```python
from build123d import *

# Parameters (mm, degrees)
BOSS_EXTRUDE1_DEPTH     = 2
BOSS_EXTRUDE2_START     = 2
BOSS_EXTRUDE2_DEPTH     = 2.5
BOSS_EXTRUDE3_START     = 4.5
SKETCH1_6_R             = 3.25
BOSS_EXTRUDE3_DEPTH     = 2
BOSS_EXTRUDE6_DEPTH     = 33.8
BOSS_EXTRUDE7_DEPTH     = 3.8
FILLET1_R               = 2
FILLET2_R               = 2
FILLET3_R               = 0.5
CUT_EXTRUDE1_REACH      = 54.552
CUT_EXTRUDE1_END_RADIUS = 27.541666667
SKETCH6_R               = 3.25


with BuildPart() as part:
    # Sketch1 → Boss-Extrude1 (new body)
    with BuildSketch(Plane(origin=(0, 0, 0), x_dir=(1, 0, 0), z_dir=(0, 1, 0))):
        with BuildLine():
            ThreePointArc((0, 8.25), (-8.25, 0), (0, -8.25))
            Line((0, -8.25), (0, -3.25))
            ThreePointArc((0, -3.25), (-3.25, 0), (0, 3.25))
            Line((0, 3.25), (0, 8.25))
        make_face()
        with BuildLine():
            Line((0, -3.25), (0, -8.25))
            ThreePointArc((0, -8.25), (5.833630945, -5.833630945), (8.25, 0))
            ThreePointArc((8.25, 0), (5.833630945, 5.833630945), (0, 8.25))
            Line((0, 8.25), (0, 3.25))
            ThreePointArc((0, 3.25), (2.298097039, 2.298097039), (3.25, 0))
            ThreePointArc((3.25, 0), (2.298097039, -2.298097039), (0, -3.25))
        make_face()
        with BuildLine():
            Line((0, -8.25), (0, -9.25))
            ThreePointArc((0, -9.25), (9.25, 0), (0, 9.25))
            Line((0, 9.25), (0, 8.25))
            ThreePointArc((0, 8.25), (5.833630945, 5.833630945), (8.25, 0))
            ThreePointArc((8.25, 0), (5.833630945, -5.833630945), (0, -8.25))
        make_face()
        with BuildLine():
            Line((0, -12.5), (22, -12.5))
            ThreePointArc((22, -12.5), (19, 0), (22, 12.5))
            Line((22, 12.5), (0, 12.5))
            Line((0, 12.5), (0, 9.25))
            ThreePointArc((0, 9.25), (9.25, 0), (0, -9.25))
            Line((0, -9.25), (0, -12.5))
        make_face()
        with BuildLine():
            Line((22, -12.5), (30, -12.5))
            Line((30, -12.5), (30, 12.5))
            Line((30, 12.5), (22, 12.5))
            ThreePointArc((22, 12.5), (19, 0), (22, -12.5))
        make_face()
    extrude(amount=BOSS_EXTRUDE1_DEPTH)

    # Sketch1<4> → Boss-Extrude2 (add)
    with BuildSketch(Plane(origin=(0, 0, 0), x_dir=(1, 0, 0), z_dir=(0, 1, 0)).offset(BOSS_EXTRUDE2_START)):
        with BuildLine():
            Line((30, -12.5), (30, 12.5))
            Line((30, 12.5), (0, 12.5))
            Line((0, 12.5), (0, 9.25))
            ThreePointArc((0, 9.25), (9.25, 0), (0, -9.25))
            Line((0, -9.25), (0, -12.5))
            Line((0, -12.5), (30, -12.5))
        make_face()
    extrude(amount=BOSS_EXTRUDE2_DEPTH)

    # Sketch1<6> → Boss-Extrude3 (add)
    with BuildSketch(Plane(origin=(0, 0, 0), x_dir=(1, 0, 0), z_dir=(0, 1, 0)).offset(BOSS_EXTRUDE3_START)):
        with BuildLine():
            Line((30, -12.5), (30, 12.5))
            Line((30, 12.5), (0, 12.5))
            Line((0, 12.5), (0, 8.25))
            ThreePointArc((0, 8.25), (-8.25, 0), (0, -8.25))
            Line((0, -8.25), (0, -12.5))
            Line((0, -12.5), (30, -12.5))
        make_face()
        with Locations(Location((0, 0, 0), (0, 0, 270))):
            Circle(SKETCH1_6_R, mode=Mode.SUBTRACT)
    extrude(amount=BOSS_EXTRUDE3_DEPTH)

    # Sketch1<8> → Boss-Extrude6 (add)
    with BuildSketch(Plane(origin=(0, 0, 0), x_dir=(1, 0, 0), z_dir=(0, 1, 0))):
        with BuildLine():
            Line((22, -12.5), (30, -12.5))
            Line((30, -12.5), (30, 12.5))
            Line((30, 12.5), (22, 12.5))
            ThreePointArc((22, 12.5), (19, 0), (22, -12.5))
        make_face()
    extrude(amount=BOSS_EXTRUDE6_DEPTH)

    # Sketch3 → Boss-Extrude7 (add)
    with BuildSketch(Plane(origin=(0, 33.8, 0), x_dir=(1, 0, 0), z_dir=(0, 1, 0))):
        with BuildLine():
            Line((11, 0), (19, 0))
            ThreePointArc((19, 0), (19.473969858, 5.087552676), (20.879566153, 10))
            Line((20.879566153, 10), (11, 0))
        make_face()
        with BuildLine():
            ThreePointArc((20.879566153, -10), (19.473969858, -5.087552676), (19, 0))
            Line((19, 0), (11, 0))
            Line((11, 0), (20.879566153, -10))
        make_face()
        with BuildLine():
            ThreePointArc((20.879566153, 10), (19.473969858, 5.087552676), (19, 0))
            ThreePointArc((19, 0), (19.473969858, -5.087552676), (20.879566153, -10))
            ThreePointArc((20.879566153, -10), (21.408679185, -11.263939941), (22, -12.5))
            Line((22, -12.5), (30, -12.5))
            Line((30, -12.5), (30, 12.5))
            Line((30, 12.5), (22, 12.5))
            ThreePointArc((22, 12.5), (21.408679185, 11.263939941), (20.879566153, 10))
        make_face()
    extrude(amount=-BOSS_EXTRUDE7_DEPTH)

    # Fillet1
    fillet1_edges = [part.edges().sort_by_distance(p)[0] for p in [
        (11, 31.9, 0),
    ]]
    fillet(fillet1_edges, radius=FILLET1_R)

    # Fillet2
    fillet2_edges = [part.edges().sort_by_distance(p)[0] for p in [
        (30, 16.9, -12.5),
        (30, 16.9, 12.5),
        (22, 20.15, -12.5),
        (22, 20.15, 12.5),
    ]]
    fillet(fillet2_edges, radius=FILLET2_R)

    # Fillet3
    fillet3_edges = [part.edges().sort_by_distance(p)[0] for p in [
        (0, 2, 8.75),
        (0, 3.25, -9.25),
        (0, 3.25, 9.25),
        (0, 2, -8.75),
        (0, 4.5, -8.75),
        (-8.25, 4.5, 0),
        (0, 4.5, 8.75),
        (-8.25, 2, 0),
    ]]
    fillet(fillet3_edges, radius=FILLET3_R)

    # Cut-Extrude1: up to this cylinder (the profile starts inside it)
    cut_extrude1_end = Plane(origin=(46.541666667, 23, 0), z_dir=(0, -1, 0)) * Cylinder(CUT_EXTRUDE1_END_RADIUS, 165.187333333, mode=Mode.PRIVATE)
    # Sketch6 → Cut-Extrude1 (cut, up to the surface)
    with BuildSketch(Plane(origin=(30, 0, 0), x_dir=(0, 0, -1), z_dir=(1, 0, 0)), mode=Mode.PRIVATE) as cut_extrude1_sk1:
        with Locations((0, 23)):
            Circle(SKETCH6_R)
    cut_extrude1_tool1 = extrude(cut_extrude1_sk1.sketch, amount=-CUT_EXTRUDE1_REACH, mode=Mode.PRIVATE) & cut_extrude1_end
    add(cut_extrude1_tool1.solids().sort_by_distance((30, 23, 0))[0], mode=Mode.SUBTRACT)


solid = part.part
```
Verification items for the finished model (mm, model axes). A direction names the side the tool comes from. Give positions to 0.01 mm unless a question says otherwise; leave off trailing zeros. Loops run counter-clockwise (first coordinate to the right, second up) from the corner with the lowest first, then second, coordinate; pieces in that order, holes last.
1. Section check B-B, the plane x = 15.5. Enter the section's corners in (y, z), then the cut area to 3 significant figures.
2. Set-up check for faces 1 (the flat face through (16.57, 31.93, 5.64)), 2 (the cylindrical face through (11.81, 31.87, -0.02)), 3 (the flat face through (0, 3, -11)): record each of +Z, -Z, +X, -X, +Y, -Y from which the full face is reachable in a straight line by a thin tool's end or side.
3. Section check C-C, the plane y = 23. Enter the section's corners in (x, z), then the cut area to 3 significant figures.
4. Thickness scan on line 1 (Y direction, x = 1, z = -4.5); line 2 (X direction, y = 6.1, z = 0); line 3 (Y direction, x = 23.5, z = 0). Record the ranges inside material, lowest first.
5. Section check D-D, the plane x = -1.5. Count the separate pieces of the cut face and the enclosed holes in it, then the cut area to 3 significant figures.
6. Go/stop test with flat-tipped pins: pin 1 Ø6 at (x, z) = (0, 0) entering from -Y; pin 2 Ø13.5 at (x, z) = (2, -3.5) entering from +Y; pin 3 Ø10 at (y, z) = (16, -9.5) entering from -X; pin 4 Ø1.3 at (y, z) = (4.5, -9.5) entering from -X. Record where each tip stops, or that it passes through.
7. Section check A-A, the plane y = 6. Enter the section's corners in (x, z), then the cut area to 3 significant figures.
Geometry says:
1. outline: (0, -12.5) - (6.5, -12.5) - (6.5, 12.5) - (0, 12.5) - close; (30, -4.55) - (33.8, -4.55) - (33.8, 4.55) - (30, 4.55) - close
1. area: 197 mm2
2. face 1: +Z, -X, +Y
2. face 2: -X, +Y
2. face 3: -Z, -X, +Y, -Y
3. outline: (19.19, -3.25) arc R27.54 ccw to (21.43, -11.32) arc R2 ccw to (23.26, -12.5) - (28, -12.5) arc R2 ccw to (30, -10.5) - (30, -3.25) - close; (19.19, 3.25) - (30, 3.25) - (30, 10.5) arc R2 ccw to (28, 12.5) - (23.26, 12.5) arc R2 ccw to (21.43, 11.32) arc R27.54 ccw to start
3. area: 177 mm2
4. line 1: y = 0 to 2, 4.5 to 6.5
4. line 2: x = -8.25 to -3.25, 3.25 to 30
4. line 3: y = 0 to 19.75, 26.25 to 33.8
5. separate pieces: 4
5. enclosed holes: 0
5. area: 41.6 mm2
6. pin 1: passes through
6. pin 2: stops at y = 6.5
6. pin 3: stops at x = 19.37
6. pin 4: stops at x = 0
7. outline: (0, -12.5) - (28, -12.5) arc R2 ccw to (30, -10.5) - (30, 10.5) arc R2 ccw to (28, 12.5) - (0, 12.5) - (0, 8.25) arc R8.25 ccw to (0, -8.25) - close; hole circle Ø6.5 at (0, 0)
7. area: 822 mm2
